The model under review builds one solid part; all positions refer to its coordinate system, in mm. A direction names the side the tool comes from. Coordinates: 2 decimals unless noted, no trailing zeros. Write each loop counter-clockwise with the first axis right and the second up, starting at its lowest first coordinate (ties: lowest second). Pieces come first, ordered by that corner, then holes.
1) Add section B-B, the plane x = -4. State the section outline as (y, z) points, then the cut area to 3 significant figures.
2) Mouldability with a two-part tool opening along Z and no side actions: class faces 1 (the cylindrical face through (-30.728, 4.056, -6.095)), 2 (the cylindrical face through (-55.99, 4.06, 37.79)), 3 (the flat face through (-8, 4, -6)), 4 (the flat face through (-48.62, 3.94, 36.36)) as released by +Z, released by -Z, zero draft, split by the parting line, or undercut.
3) Add section A-A, the plane z = 27.5. State the section outline as (x, y) points, then the cut area to 3 significant figures.
4) Add section C-C, the plane y = 4.5. Give the number of separate pieces and of enclosed holes in the cut face, then the cut area to 3 significant figures.
5) For P1, Ø4, axis at y = 4, z = 48, coming from the -X side; P2, Ø4, axis at x = -26, y = 3, coming from the -Z side; P3, Ø2.5, axis at x = -3, y = 3, coming from the +Z side, all flat-tipped, find the tip position at first contact; note any pin that passes through.
6) Machinability: for faces 5 (the flat face through (0, 4, 29)), 6 (the flat face through (-33, 0, 40)), 7 (the cylindrical face through (-33.138, 4.056, 42.502)), which of the approach directions +Z, -Z, +X, -X, +Y, -Y give a long, thin tool a straight path to every point of the face, cutting with its end or side? Answer none if there is none.
7) Add section D-D, the plane z = 72. State the section outline as (x, y) points, then the cut area to 3 significant figures.
8) For line 1 (Z direction, x = -10.5, y = 6); line 2 (Z direction, x = -23, y = 2); line 3 (X direction, y = 2.75, z = 21.5), list the stretches that pass through material, from the lowest coordinate up.
from build123d import *

# Parameters (mm, degrees)
BOSS_EXTRUDE1_DEPTH = 8
SKETCH2_W           = 16
SKETCH2_H           = 9
SKETCH2_W_2         = 10
SKETCH2_H_2         = 3
SKETCH2_W_3         = 9
SKETCH2_H_3         = 16
SKETCH2_W_4         = 3
SKETCH2_H_4         = 10
BOSS_EXTRUDE2_DEPTH = 8
FILLET1_R           = 3


with BuildPart() as part:
    # Sketch1 → Boss-Extrude1 (new body)
    with BuildSketch(Plane(origin=(0, 0, 0), x_dir=(1, 0, 0), z_dir=(0, 1, 0))):
        Polygon((-25, 0), (0, 0), (0, -80), (-33, -80), (-53.047096556, -45.386217778), (-39.710857444, -38.520016036), (-39.710857444, -8.520016036), align=None)
        Polygon((-23.119252614, -7), (-7, -7), (-7, -73), (-28.964892735, -73), (-43.303341696, -48.242901217), (-32.710857444, -42.789329696), (-32.710857444, -12.555123301), align=None, mode=Mode.SUBTRACT)
    extrude(amount=BOSS_EXTRUDE1_DEPTH)

    # Sketch2 → Boss-Extrude2 (add)
    # profile 1 of 5: a face of its own
    with BuildSketch(Plane(origin=(0, 0, 0), x_dir=(1, 0, 0), z_dir=(0, 1, 0))):
        Polygon((-53.047096556, -45.386217778), (-38.821774837, -38.062269253), (-42.941495882, -30.060525786), (-57.166817601, -37.384474311), align=None)
        Polygon((-51.753089082, -41.345729608), (-42.862263008, -36.768261779), (-44.235503356, -34.101013957), (-53.12632943, -38.678481785), align=None, mode=Mode.SUBTRACT)
    # profile 2 of 5: a face of its own
    with BuildSketch(Plane(origin=(0, 0, 0), x_dir=(1, 0, 0), z_dir=(0, 1, 0))):
        Polygon((-39.710857444, -8.520016036), (-25.865344556, -0.501177414), (-30.375941281, 7.286923586), (-44.221454169, -0.731915036), align=None)
        Polygon((-38.618356019, -4.420450128), (-29.964910464, 0.591324011), (-31.468442706, 3.187357678), (-40.121888261, -1.824416461), align=None, mode=Mode.SUBTRACT)
    # profile 3 of 5: a face of its own
    with BuildSketch(Plane(origin=(0, 0, 0), x_dir=(1, 0, 0), z_dir=(0, 1, 0))):
        with Locations((-8, 4.5)):
            Rectangle(SKETCH2_W, SKETCH2_H)
        with Locations((-8, 4.5)):
            Rectangle(SKETCH2_W_2, SKETCH2_H_2, mode=Mode.SUBTRACT)
    # profile 4 of 5: a face of its own
    with BuildSketch(Plane(origin=(0, 0, 0), x_dir=(1, 0, 0), z_dir=(0, 1, 0))):
        with Locations((-25, -84.5)):
            Rectangle(SKETCH2_W, SKETCH2_H)
        with Locations((-25, -84.5)):
            Rectangle(SKETCH2_W_2, SKETCH2_H_2, mode=Mode.SUBTRACT)
    # profile 5 of 5: a face of its own
    with BuildSketch(Plane(origin=(0, 0, 0), x_dir=(1, 0, 0), z_dir=(0, 1, 0))):
        with Locations((4.5, -72)):
            Rectangle(SKETCH2_W_3, SKETCH2_H_3)
        with Locations((4.5, -72)):
            Rectangle(SKETCH2_W_4, SKETCH2_H_4, mode=Mode.SUBTRACT)
    extrude(amount=BOSS_EXTRUDE2_DEPTH)

    # Fillet1
    fillet1_edges = [part.edges().sort_by_distance(p)[0] for p in [
        (0, 4, -9),
        (-16, 4, -9),
        (9, 4, 64),
        (9, 4, 80),
        (-32.710857444, 4, 42.789329696),
        (-42.941495882, 4, 30.060525786),
        (-57.166817601, 4, 37.384474311),
        (-30.375941281, 4, -7.286923586),
        (-44.221454169, 4, 0.731915036),
        (-17, 4, 89),
        (-33, 4, 89),
    ]]
    fillet(fillet1_edges, radius=FILLET1_R)


solid = part.part
Geometry results:
1. outline: (0, -9) - (8, -9) - (8, -6) - (0, -6) - close; (0, -3) - (8, -3) - (8, 80) - (0, 80) - close
1. area: 688 mm2
2. face 1: released by -Z
2. face 2: split by the parting line
2. face 3: undercut
2. face 4: undercut
3. outline: (-39.71, 0) - (-32.71, 0) - (-32.71, 8) - (-39.71, 8) - close; (-7, 0) - (0, 0) - (0, 8) - (-7, 8) - close
3. area: 112 mm2
4. separate pieces: 1
4. enclosed holes: 6
4. area: 2,040 mm2
5. P1: stops at x = -52.69
5. P2: stops at z = -3.18
5. P3: stops at z = 80
6. face 5: -Z, +X, +Y, -Y
6. face 6: +Z, -Z, +X, -X, -Y
6. face 7: +Y, -Y
7. outline: (-37.63, 0) - (-29.54, 0) - (-29.54, 8) - (-37.63, 8) - close; (-7, 0) - (3, 0) - (3, 8) - (-7, 8) - close; (6, 0) - (9, 0) - (9, 8) - (6, 8) - close
7. area: 169 mm2
8. line 1: z = -9 to -6, -3 to 7, 73 to 80
8. line 2: z = 0 to 7, 73 to 83, 86 to 89
8. line 3: x = -39.71 to -32.71, -7 to 0
